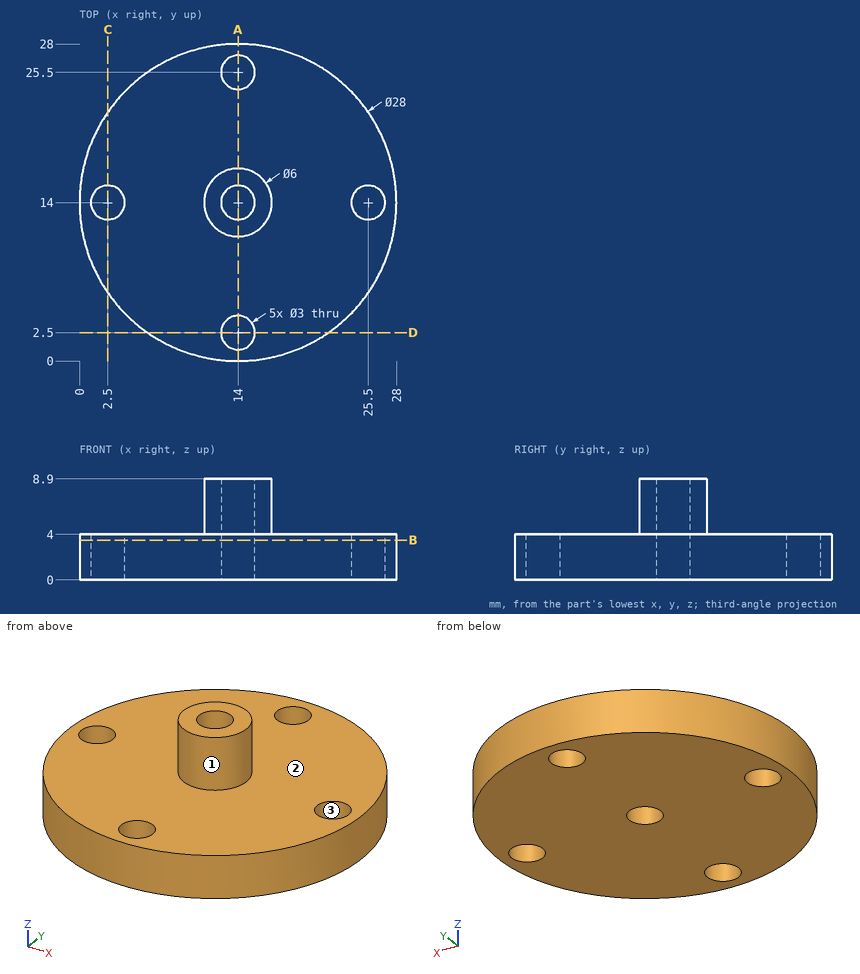
Can you work these out from the drawing? Everything is in mm from the part's minimum corner. Give positions to 0.01 mm unless a question says otherwise; leave off trailing zeros. Loops run counter-clockwise (first coordinate to the right, second up) from the corner with the lowest first, then second, coordinate; pieces in that order, holes last. Notation, with made-up numbers: (82.5, 73.25) -> (92.5, 73.25) arc R21 cw to (92.5, 100.25) -> close; hole circle Ø11 at (39.5, 81). An arc over 180 degrees is marked (long way). Return JSON: item names as keys, results as strings.
Q1. I want a section at B-B, the plane z = 3.5. List the corners of the cut face in (x, y) for me.
Checks:
{"outline": "circle Ø28 at (14, 14); hole circle Ø3 at (2.5, 14); hole circle Ø3 at (14, 2.5); hole circle Ø3 at (14, 14); hole circle Ø3 at (14, 25.5); hole circle Ø3 at (25.5, 14)"}
Q2. I need wall thicknesses on probe 1 along Y at (x, z) = (14, 2.2); probe 2 along Z at (x, y) = (22, 5.75); probe 3 along Y at (x, z) = (2.5, 1.65). Which ranges of each line are inside material? Lowest first, please.
Checks:
{"probe 1": "y = 0 to 1, 4 to 12.5, 15.5 to 24, 27 to 28", "probe 2": "z = 0 to 4", "probe 3": "y = 6.02 to 12.5, 15.5 to 21.98"}
Q3. For pin 1 Ø5 at (x, y) = (14, 2.5) entering from +Z; pin 2 Ø14 at (x, y) = (17, 13.5) entering from +Z; pin 3 Ø5 at (y, z) = (20.5, 1) entering from +X, each with a flat end and sliding along its axis, tell me the tip position at first contact or that it passes through.
Checks:
{"pin 1": "stops at z = 4", "pin 2": "stops at z = 8.9", "pin 3": "stops at x = 27.42"}
Q4. I want a section at C-C, the plane x = 2.5. List the corners of the cut face in (y, z) for me, then the cut area to 3 significant figures.
Checks:
{"outline": "(6.02, 0) -> (12.5, 0) -> (12.5, 4) -> (6.02, 4) -> close; (15.5, 0) -> (21.98, 0) -> (21.98, 4) -> (15.5, 4) -> close", "area": "51.9 mm2"}
Q5. I want a section at A-A, the plane x = 14. List the corners of the cut face in (y, z) for me.
Checks:
{"outline": "(0, 0) -> (1, 0) -> (1, 4) -> (0, 4) -> close; (4, 0) -> (12.5, 0) -> (12.5, 8.9) -> (11, 8.9) -> (11, 4) -> (4, 4) -> close; (15.5, 0) -> (24, 0) -> (24, 4) -> (17, 4) -> (17, 8.9) -> (15.5, 8.9) -> close; (27, 0) -> (28, 0) -> (28, 4) -> (27, 4) -> close"}
Q6. We'd pull the mould along Y, two halves only. Please class the marked faces 1, 2 and 3: released by +Y, released by -Y, zero draft, split by the parting line, or undercut.
Checks:
{"face 1": "split by the parting line", "face 2": "zero draft", "face 3": "undercut"}
